Could you check a few things on this model? Use its own coordinates, in mm. Face numbers are marked on the shaded views. A direction names the side the tool comes from. Give positions to 0.01 mm unless a question says otherwise; leave off trailing zeros. Loops run counter-clockwise (first coordinate to the right, second up) from the corner with the lowest first, then second, coordinate; pieces in that order, holes last. Notation, with made-up numbers: (-34.75, -23.75) -> (-2.75, -23.75) arc R27 ccw to (-2.75, 13.25) -> close; hole circle Ø7 at (37, -29.5). An arc over 180 degrees is marked (long way). Write item = value, one per line. Start each with the question number.
1) I need wall thicknesses on probe 1 along Z at (x, y) = (0, 1.45); probe 2 along X at (y, z) = (1.5, -2); probe 3 along Y at (x, z) = (4.75, 1.75). Which ranges of each line are inside material? Lowest first, please. Write a range as from..to.
2) I want a section at A-A (x = 0). List the corners of the cut face in (y, z) for me.
3) I want a section at D-D (y = 24.75). List the corners of the cut face in (x, z) for me, and give its area (3 significant figures).
4) I'm going to push flat-ended pins straight in: pin 1 Ø1.5 at (x, z) = (-2.5, 4.5) entering from +Y; pin 2 Ø3 at (x, y) = (0, 4.5) entering from +Z; pin 3 Ø4 at (x, z) = (-2, -0.5) entering from -Y; pin 4 Ø1.5 at (x, y) = (0.5, 26) entering from -Z. Where does each tip first touch, or does it pass through?
5) I want a section at B-B (z = 0). List the corners of the cut face in (x, y) for me, and give its area (3 significant figures).
6) If we mould it in two halves opening along X, with no side actions, what happens to the marked faces 6, 7, 8 and 9? For each: +X half, -X half, draft (parallel to the pull), parting line (faces both ways), or undercut.
7) On a 3-axis mill with a long thin cutter (end or side, diameter ignored), from which of +Z, -Z, +X, -X, +Y, -Y can I reach the whole of each face in a straight line? I mean the marked faces 1, 2, 3, 4 and 5. Say none if no direction works.
8) I want a section at C-C (y = 12.25). List the corners of the cut face in (x, z) for me, and give its area (3 significant figures).
from build123d import *

# Parameters (mm, degrees)
F0_R     = 7
F1_DEPTH = 2
F2_R     = 5.75
F3_DEPTH = 21
F4_R     = 3
F5_DEPTH = 20
F6_R     = 6.25
F6_R_2   = 4.5
F7_DEPTH = 1.9
F8_W     = 5
F8_H     = 8
F9_DEPTH = 0.3


with BuildPart() as f1:
    # F0 (on Front) → F1 (new body)
    with BuildSketch(Plane.XZ):
        Circle(F0_R)
    extrude(amount=-F1_DEPTH)

    # F2 (on face) → F3 (join)
    with BuildSketch(Plane(origin=(0, 2, 0), x_dir=(-1, 0, 0), z_dir=(0, 1, 0))):
        Circle(F2_R)
    extrude(amount=F3_DEPTH)

    # F4 (on face) → F5 (cut)
    with BuildSketch(Plane.XZ):
        Circle(F4_R)
    extrude(amount=-F5_DEPTH, mode=Mode.SUBTRACT)

    # F6 (on face) → F7 (cut)
    with BuildSketch(Plane.XZ):
        Circle(F6_R)
        Circle(F6_R_2, mode=Mode.SUBTRACT)
    extrude(amount=-F7_DEPTH, mode=Mode.SUBTRACT)

    # F8 (on Top) → F9 (join, symmetric)
    with BuildSketch(Plane.XY):
        with Locations((0, 26)):
            Rectangle(F8_W, F8_H)
    extrude(amount=F9_DEPTH, both=True)


solid = f1.part
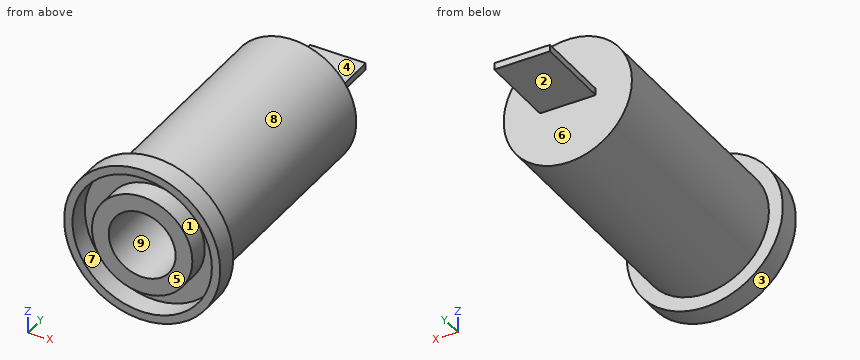
Answer list:
q1.probe_1 = -7..-6.25, -4.5..-3, 3..4.5, 6.25..7
q1.probe_2 = -6.71..-5.92, -4.03..-2.24, 2.24..4.03, 5.92..6.71
q1.probe_3 = 1.9..23
q2.outline = (0, -7) -> (2, -7) -> (2, -5.75) -> (23, -5.75) -> (23, -0.3) -> (30, -0.3) -> (30, 0.3) -> (23, 0.3) -> (23, 5.75) -> (2, 5.75) -> (2, 7) -> (0, 7) -> (0, 6.25) -> (1.9, 6.25) -> (1.9, 4.5) -> (0, 4.5) -> (0, 3) -> (20, 3) -> (20, -3) -> (0, -3) -> (0, -4.5) -> (1.9, -4.5) -> (1.9, -6.25) -> (0, -6.25) -> close
q3.outline = (-2.5, -0.3) -> (2.5, -0.3) -> (2.5, 0.3) -> (-2.5, 0.3) -> close
q3.area = 3.00 mm^2
q4.pin_1 = 23
q4.pin_2 = 5.75
q4.pin_3 = 0
q4.pin_4 = -0.3
q5.outline = (-7, 0) -> (-6.25, 0) -> (-6.25, 1.9) -> (-4.5, 1.9) -> (-4.5, 0) -> (-3, 0) -> (-3, 20) -> (3, 20) -> (3, 0) -> (4.5, 0) -> (4.5, 1.9) -> (6.25, 1.9) -> (6.25, 0) -> (7, 0) -> (7, 2) -> (5.75, 2) -> (5.75, 23) -> (2.5, 23) -> (2.5, 30) -> (-2.5, 30) -> (-2.5, 23) -> (-5.75, 23) -> (-5.75, 2) -> (-7, 2) -> close
q5.area = 178 mm^2
q6.face_6 = draft
q6.face_7 = undercut
q6.face_8 = parting line
q6.face_9 = undercut
q7.face_1 = -Y
q7.face_2 = -Z, +X, -X, +Y
q7.face_3 = +Y, -Y
q7.face_4 = +Z, +X, -X, +Y
q7.face_5 = +Z, -Z, +X, -X, -Y
q8.outline = circle Ø11.5 at (0, 0); hole circle Ø6 at (0, 0)
q8.area = 75.6 mm^2
